The listing builds one solid part. Answer for the finished solid, in the listing's coordinates (mm). A direction names the side the tool comes from. Give positions to 0.01 mm unless a question says otherwise; leave off trailing zeros. Write each loop counter-clockwise with the first axis right and the second up, starting at its lowest first coordinate (ties: lowest second). Pieces come first, ordered by that corner, then holes. Notation, with made-up numbers: (-24.5, -7.75) -> (-19.5, -7.75) arc R8 cw to (-19.5, -1.75) -> close; hole circle Ø3 at (81.5, 72). An arc over 180 degrees is marked (long way). One line per question, with ' | ' between items.
from build123d import *

# Parameters (mm, degrees)
F1_DEPTH = 15
F2_R     = 4.6736
F3_DEPTH = 29.8
F4_R     = 1


with BuildPart() as f1:
    # F0 (on Front) → F1 (new body)
    with BuildSketch(Plane.XZ):
        with BuildLine():
            ThreePointArc((-1.364345, -5.328092), (0.234996, 5.494977), (0.904479, -5.425119))
            Line((0.904479, -5.425119), (0.904479, -26.600169))
            Line((0.904479, -26.600169), (3.904479, -26.600169))
            Line((3.904479, -26.600169), (3.904479, -7.550169))
            ThreePointArc((3.904479, -7.550169), (0.2632, 8.495924), (-4.364345, -7.294004))
            Line((-4.364345, -7.294004), (-4.364345, -26.344004))
            Line((-4.364345, -26.344004), (-1.364345, -26.344004))
            Line((-1.364345, -26.344004), (-1.364345, -5.328092))
        make_face()
    extrude(amount=F1_DEPTH)

    # F2 (on face) → F3 (cut, symmetric)
    with BuildSketch(Plane.YZ.offset(3.904479)):
        with Locations((-7.5, -16.32629)):
            Circle(F2_R)
    extrude(amount=F3_DEPTH, both=True, mode=Mode.SUBTRACT)

    # F4
    f4_edges = [f1.edges().sort_by_distance(p)[0] for p in [
        (-4.364345, 0, -16.819004),
        (0.2632, 0, 8.495924),
        (3.904479, 0, -17.075169),
        (2.404479, 0, -26.600169),
        (-2.864345, 0, -26.344004),
        (3.904479, -7.5, -26.600169),
        (-4.364345, -7.5, -26.344004),
    ]]
    fillet(f4_edges, radius=F4_R)


solid = f1.part
Item 1: Find section C-C (y = -1.75). Write down the section's boundary in (x, z), then the cut area to 3 significant figures.
Answers below:
outline: (-4.36, -25.34) arc R1 ccw to (-3.36, -26.34) -> (-1.36, -26.34) -> (-1.36, -5.33) arc R5.5 cw (long way) to (0.9, -5.43) -> (0.9, -26.6) -> (2.9, -26.6) arc R1 ccw to (3.9, -25.6) -> (3.9, -7.55) arc R8.5 ccw (long way) to (-4.36, -7.29) -> close | area: 235 mm²
Item 2: Find section A-A (y = -7.5). Write down the section's boundary in (x, z), then the cut area to 3 significant figures.
Answers below:
outline: (-4.36, -25.34) arc R1 ccw to (-3.36, -26.34) -> (-1.36, -26.34) -> (-1.36, -21) -> (-4.36, -21) -> close; (-4.36, -11.65) -> (-1.36, -11.65) -> (-1.36, -5.33) arc R5.5 cw (long way) to (0.9, -5.43) -> (0.9, -11.65) -> (3.9, -11.65) -> (3.9, -7.55) arc R8.5 ccw (long way) to (-4.36, -7.29) -> close; (0.9, -26.6) -> (2.9, -26.6) arc R1 ccw to (3.9, -25.6) -> (3.9, -21) -> (0.9, -21) -> close | area: 179 mm²
Item 3: A tool of negligible diameter and unlimited length cuts with its end or side. For faces 4 (the face through (0.904, -7, -11)), 5 (the face through (3.604, -0.285, -16.127)), 6 (the face through (-4.064, -0.285, -16.154)), 7 (the face through (-4.364, -13, -16)), from which of +Z, -Z, +X, -X, +Y, -Y can it reach the whole face along a straight path? Write none if from no direction.
Answers below:
face 4: -Z, +Y, -Y | face 5: -Z, +X, +Y | face 6: -Z, -X, +Y | face 7: -Z, -X, +Y, -Y
Item 4: Flat-ended cylindrical pins translate along their axes: pin 1 (6 mm diameter, centred on x = -5.5, z = -4.5, fed in from +Y); pin 2 (7.5 mm diameter, centred on y = -10.5, z = -11.5, fed in from +X); pin 3 (1 mm diameter, centred on x = -1, y = -5, fed in from -Z); pin 4 (1.5 mm diameter, centred on x = -4.5, y = -9.5, fed in from +Z). Find the tip coordinate at first contact, or state that the pin passes through.
Answers below:
pin 1: y = 0 | pin 2: x = 3.9 | pin 3: z = -26.34 | pin 4: z = 7.63
Item 5: Find section D-D (x = -1.75). Count the separate pieces of the cut face and the enclosed holes in it, then the cut area to 3 significant figures.
Answers below:
separate pieces: 2 | enclosed holes: 1 | area: 294 mm²
Item 6: Determine the mould class of faces 1 (the face through (-2.843, -8.108, -11.692)), 2 (the face through (-1.364, -7, -11)), 3 (the face through (3.904, -9, -21)) for opening direction X: pulls with the +X half, pulls with the -X half, needs draft (parallel to the pull), parting line crosses it, or undercut.
Answers below:
face 1: needs draft | face 2: undercut | face 3: pulls with the +X half
Item 7: Consider line 1 (Z direction, x = 1.95, y = -7.5); line 2 (Z direction, x = 2.85, y = -7.5); line 3 (X direction, y = -3.25, z = -8). Determine where each line is inside the solid, lowest interval first. Write a range as [from, to].
Answers below:
line 1: [-26.6, -21], [-11.65, -5.14], [5.14, 8.27] | line 2: [-26.6, -21], [-11.65, -4.7], [4.7, 8.01] | line 3: [-4.36, -1.36], [0.9, 3.9]
Item 8: Find section B-B (z = -17). Write down the section's boundary in (x, y).
Answers below:
outline: (-4.36, -15) -> (-1.36, -15) -> (-1.36, -12.12) -> (-4.36, -12.12) -> close; (-4.36, -2.88) -> (-1.36, -2.88) -> (-1.36, 0) -> (-3.36, 0) arc R1 ccw to (-4.36, -1) -> close; (0.9, -15) -> (3.9, -15) -> (3.9, -12.12) -> (0.9, -12.12) -> close; (0.9, -2.88) -> (3.9, -2.88) -> (3.9, -1) arc R1 ccw to (2.9, 0) -> (0.9, 0) -> close
